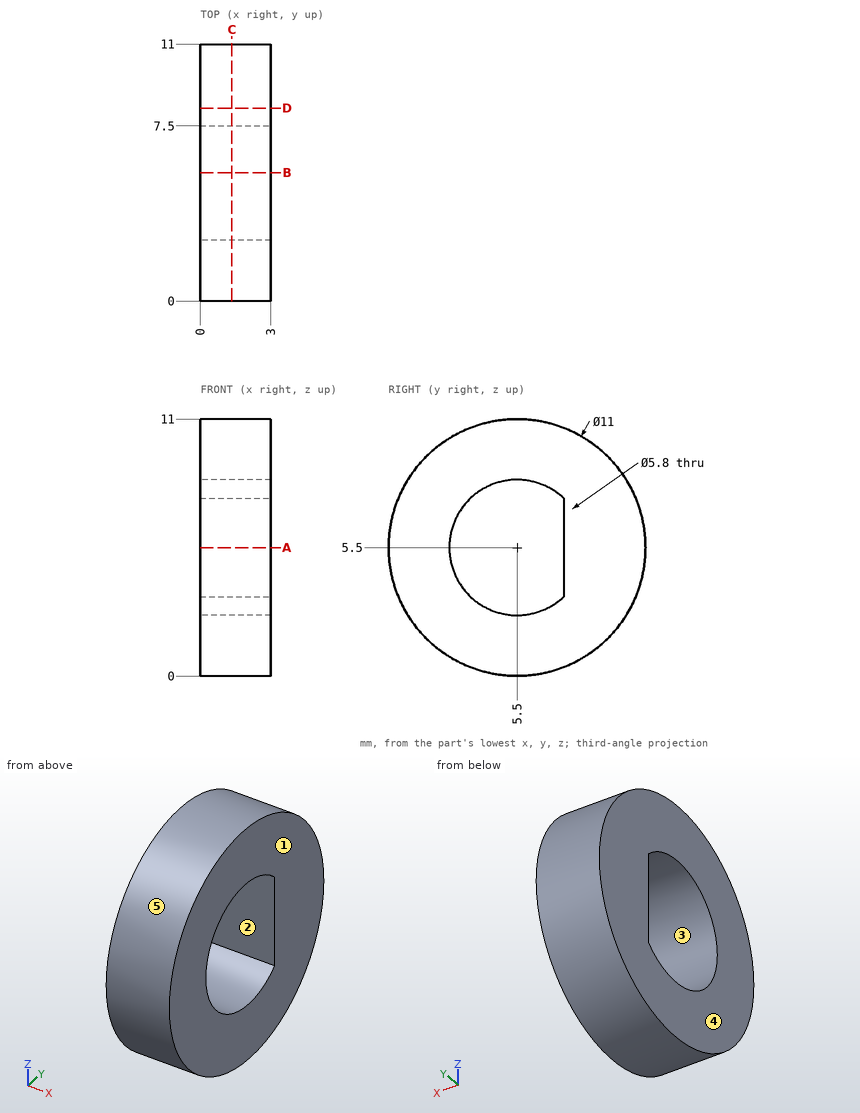
Print and shaded views of the part. All mm, measured from the part's lowest x, y and z. A direction names the side the tool comes from. Coordinates: 2 decimals unless noted, no trailing zeros. Loops run counter-clockwise (first coordinate to the right, second up) from the corner with the lowest first, then second, coordinate; pieces in that order, holes last. Notation, with made-up numbers: (-28, -3.5) -> (15, -3.5) arc R21 cw to (15, 34.5) -> close; hole circle Ø3 at (-23.5, -4.75). An arc over 180 degrees is marked (long way). Use one line per item in the form item = value. Start each with the question number.
(1) Cut at D-D on y = 8.25. Give the cut face in (x, z), and give its area (3 significant figures).
(2) Cut at C-C on x = 1.35. Give the cut face in (y, z).
(3) Cut at B-B on y = 5.5. Give the cut face in (x, z), and give its area (3 significant figures).
(4) Probe probe 1 along Z at (x, y) = (0.7, 5.5); probe 2 along Z at (x, y) = (1.95, 7.25); probe 3 along Y at (x, z) = (1.8, 6). List the from-to ranges inside material, lowest first. Write a range as from..to.
(5) Tool access for the marked faces 1 and 2: list every direction of +Z, -Z, +X, -X, +Y, -Y with a clear straight run to the whole face (end or side of a thin tool).
(6) Cut at A-A on z = 5.5. Give the cut face in (x, y), and give its area (3 significant figures).
(7) Pull direction Y, two halves, no side cores. Call the marked faces 3, 4 and 5: pulls with the +Y half, pulls with the -Y half, needs draft (parallel to the pull), parting line crosses it, or undercut.
(8) Flat gauge pins, fed straight in: pin 1 (1 mm diameter, centred on x = 0.5, y = 9, fed in from +Z); pin 2 (1.5 mm diameter, centred on x = 1, z = 4.5, fed in from -Y). Where does each tip first touch, or does it go through?
Values:
q1.outline = (0, 0.74) -> (3, 0.74) -> (3, 10.26) -> (0, 10.26) -> close
q1.area = 28.6 mm2
q2.outline = circle Ø11 at (5.5, 5.5); hole (7.5, 3.4) -> (7.5, 7.6) arc R2.9 ccw (long way) to start
q3.outline = (0, 0) -> (3, 0) -> (3, 2.6) -> (0, 2.6) -> close; (0, 8.4) -> (3, 8.4) -> (3, 11) -> (0, 11) -> close
q3.area = 15.6 mm2
q4.probe_1 = 0..2.6, 8.4..11
q4.probe_2 = 0.29..3.19, 7.81..10.71
q4.probe_3 = 0.02..2.64, 7.5..10.98
q5.face_1 = +Z, -Z, +X, +Y, -Y
q5.face_2 = +X, -X
q6.outline = (0, 0) -> (3, 0) -> (3, 2.6) -> (0, 2.6) -> close; (0, 7.5) -> (3, 7.5) -> (3, 11) -> (0, 11) -> close
q6.area = 18.3 mm2
q7.face_3 = undercut
q7.face_4 = needs draft
q7.face_5 = parting line crosses it
q8.pin_1 = 10.11
q8.pin_2 = 0.01
